```python
from build123d import *

# Parameters (mm, degrees)
PAD077_DEPTH            = 11.5
SKETCH069_W             = 10.25
SKETCH069_H             = 30
PAD078_DEPTH            = 3
SKETCH070_R             = 2.75
POCKET048_DEPTH         = 5
SKETCH148_W             = 4
SKETCH148_H             = 20
POCKET049_DEPTH         = 11.501
POCKET049_DEPTH_BACK    = 11.501
SKETCH149_W             = 20
SKETCH149_H             = 4
PAD079_DEPTH            = 23
SKETCH150_R             = 2.75
POCKET050_DEPTH         = 34.001
FILLET003_R             = 9
BODY057_PLACEMENT_ANGLE = 90


with BuildPart() as part:
    # Sketch068 → Pad077 (new body, symmetric)
    with BuildSketch(Plane.XY):
        Polygon((0, 0), (10.25, 0), (10.25, 20), (14.25, 20), (14.25, -34), (10.25, -34), (10.25, -4), (0, -4), align=None)
    pad077 = extrude(amount=PAD077_DEPTH, both=True)

    # Sketch069 (on Face9 of Pad043) → Pad078 (join)
    with BuildSketch(Plane(origin=(0, 0, -11.5), x_dir=(1, 0, 0), z_dir=(0, 0, -1))):
        with Locations((5.125, 19)):
            Rectangle(SKETCH069_W, SKETCH069_H)
    pad078 = extrude(amount=-PAD078_DEPTH)

    # Sketch070 (on Face9 of Pad044) → Pocket048 (cut)
    with BuildSketch(Plane.YZ.offset(14.25)):
        with Locations((-25, 0)):
            Circle(SKETCH070_R)
        with Locations((10, 0)):
            Circle(SKETCH070_R)
    pocket048 = extrude(amount=-POCKET048_DEPTH, mode=Mode.SUBTRACT)

    # Mirrored028: Pad077, Pad078, Pocket048 across Sketch068 V_Axis
    add(pad077.mirror(Plane(origin=(0, 0, 0), x_dir=(0, 0, 1), z_dir=(1, 0, 0))))
    add(pad078.mirror(Plane(origin=(0, 0, 0), x_dir=(0, 0, 1), z_dir=(1, 0, 0))))
    add(pocket048.mirror(Plane(origin=(0, 0, 0), x_dir=(0, 0, 1), z_dir=(1, 0, 0))), mode=Mode.SUBTRACT)

    # Sketch148 → Pocket049 (cut, two sides)
    with BuildSketch(Plane.XY) as pocket049_sk:
        with Locations((-12.25, 10)):
            Rectangle(SKETCH148_W, SKETCH148_H)
    extrude(amount=-POCKET049_DEPTH, mode=Mode.SUBTRACT)
    extrude(pocket049_sk.sketch, amount=POCKET049_DEPTH_BACK, mode=Mode.SUBTRACT)

    # Sketch149 → Pad079 (join)
    with BuildSketch(Plane.XY.offset(-11.5)):
        with Locations((0, -2)):
            Rectangle(SKETCH149_W, SKETCH149_H)
    extrude(amount=-PAD079_DEPTH)

    # Sketch150 → Pocket050 (cut, through all)
    with BuildSketch(Plane(origin=(0, 0, -23), x_dir=(1, 0, 0), z_dir=(0, -1, 0))):
        Circle(SKETCH150_R)
    extrude(amount=POCKET050_DEPTH, mode=Mode.SUBTRACT)

    # Fillet003
    fillet003_edges = [part.edges().sort_by_distance(p)[0] for p in [
        (10, -2, -34.5),
        (-10, -2, -34.5),
    ]]
    fillet(fillet003_edges, radius=FILLET003_R)


with BuildPart() as part_1:
    # Body057 placement: moved
    add(part.part.moved(Location((-138.5, 0, 0))).rotate(Axis((-138.5, 0, 0), (0, 0, 1)), BODY057_PLACEMENT_ANGLE))


solid = part_1.part
```
Verification items for the finished model (mm, model axes). A direction names the side the tool comes from. Coordinates: 2 decimals unless noted, no trailing zeros. Loops run counter-clockwise (first coordinate to the right, second up) from the corner with the lowest first, then second, coordinate; pieces in that order, holes last. Notation, with made-up numbers: (-32, 28) - (1, 28) arc R21 ccw to (1, 61) - close; hole circle Ø7 at (36.5, 35.5). An arc over 180 degrees is marked (long way). Return JSON: item names as keys, results as strings.
1. Section check A-A, the plane y = 0. Record the boundary of the cut face in (x, z), then the cut area to 3 significant figures.
Established:
{"outline": "(-138.5, -34.5) - (-134.5, -34.5) - (-134.5, -25.75) - (-138.5, -25.75) - close; (-138.5, -20.25) - (-134.5, -20.25) - (-134.5, -11.5) - (-104.5, -11.5) - (-104.5, -8.5) - (-134.5, -8.5) - (-134.5, 11.5) - (-138.5, 11.5) - close", "area": "252 mm2"}
2. Section check B-B, the plane x = -113.5. Record the boundary of the cut face in (y, z).
Established:
{"outline": "(-14.25, -11.5) - (14.25, -11.5) - (14.25, -2.75) - (10.25, -2.75) - (10.25, -8.5) - (-10.25, -8.5) - (-10.25, -2.75) - (-14.25, -2.75) - close; (-14.25, 2.75) - (-10.25, 2.75) - (-10.25, 11.5) - (-14.25, 11.5) - close; (10.25, 2.75) - (14.25, 2.75) - (14.25, 11.5) - (10.25, 11.5) - close"}
3. Mould release check, pull along X, two halves, no side actions. Record for faces 1 (the flat face through (-119, 0, -11.5)), 2 (the flat face through (-104.5, 1, -9)), 3 (the cylindrical face through (-151.12, 12.28, 0.83)): +X half, -X half, draft (parallel to the pull), parting line (faces both ways), or undercut.
Established:
{"face 1": "draft", "face 2": "+X half", "face 3": "undercut"}
4. Thickness scan on L1, parallel to Z at x = -136.5, y = 0; L2, parallel to Z at x = -148.5, y = 11.6; L3, parallel to Y at x = -132, z = 1. Record the ranges inside material, lowest first.
Established:
{"L1": "z = -34.5 to -25.75, -20.25 to 11.5", "L2": "z = -11.5 to -2.75, 2.75 to 11.5", "L3": "y = -14.25 to -10.25, 10.25 to 14.25"}
5. Section check C-C, the plane z = -23. Record the boundary of the cut face in (x, y).
Established:
{"outline": "(-138.5, -10) - (-134.5, -10) - (-134.5, -2.75) - (-138.5, -2.75) - close; (-138.5, 2.75) - (-134.5, 2.75) - (-134.5, 10) - (-138.5, 10) - close"}
6. Tool access check on faces 4 (the flat face through (-134.5, -2, -20)), 5 (the flat face through (-134.5, 0, 2)), 6 (the flat face through (-138.5, -2, -11)). Record the directions out of +Z, -Z, +X, -X, +Y, -Y that give a thin tool (end or side, any length) a straight path to the whole face; none if there is none.
Established:
{"face 4": "-Z, +X, +Y, -Y", "face 5": "+Z, +X", "face 6": "+Z, -Z, -X, -Y"}
7. Go/stop test with flat-tipped pins: pin 1 (10 mm diameter, centred on y = -3.5, z = -21.5, fed in from -X); pin 2 (12 mm diameter, centred on x = -133.5, y = -10, fed in from -Z); pin 3 (6 mm diameter, centred on x = -147, z = 1, fed in from -Y). Record where each tip stops, or that it passes through.
Established:
{"pin 1": "stops at x = -138.5", "pin 2": "stops at z = -33.96", "pin 3": "stops at y = 10.25"}
8. Section check D-D, the plane x = -148.5. Record the boundary of the cut face in (y, z), then the cut area to 3 significant figures.
Established:
{"outline": "(10.25, -11.5) - (14.25, -11.5) - (14.25, -2.75) - (10.25, -2.75) - close; (10.25, 2.75) - (14.25, 2.75) - (14.25, 11.5) - (10.25, 11.5) - close", "area": "70.0 mm2"}
